Print and shaded views of the part. All mm, measured from the part's lowest x, y and z. A direction names the side the tool comes from. Round coordinates to 2 decimals unless told otherwise and drop trailing zeros. Loops run counter-clockwise (first coordinate to the right, second up) from the corner with the lowest first, then second, coordinate; pieces in that order, holes last. Notation, with made-up numbers: (72.25, 25.5) - (100.25, 25.5) arc R17 cw to (100.25, 45.5) - close; hole circle Ø3 at (48.25, 83). An arc over 180 degrees is marked (long way). Use one line per item in the form item = value. Start each with the question number.
Q1. Saw through at D-D (z = 5.25). Give the cut face in (x, y), then the cut area to 3 significant figures.
Q2. Pin check, flat tips, straight feed: pin 1 (4 mm diameter, centred on y = 8.5, z = 6, fed in from +X); pin 2 (1 mm diameter, centred on x = 9.5, z = 11.5, fed in from +Y). Stop position of each tip, or through.
Q3. Drill centre lines: line 1 (Y direction, x = 0.35, z = 7.5); line 2 (Y direction, x = 12.75, z = 1.5). Where is each one in solid material? Low to high.
Q4. 3-axis set-ups, long thin cutter, end or side, ignore diameter. For the marked faces 1 and 2: which of +Z, -Z, +X, -X, +Y, -Y reach the whole face in a straight line?
Q5. Saw through at A-A (y = 7.5). Give the cut face in (x, z), then the cut area to 3 significant figures.
Q6. Saw through at B-B (z = 7.5). Give the cut face in (x, y).
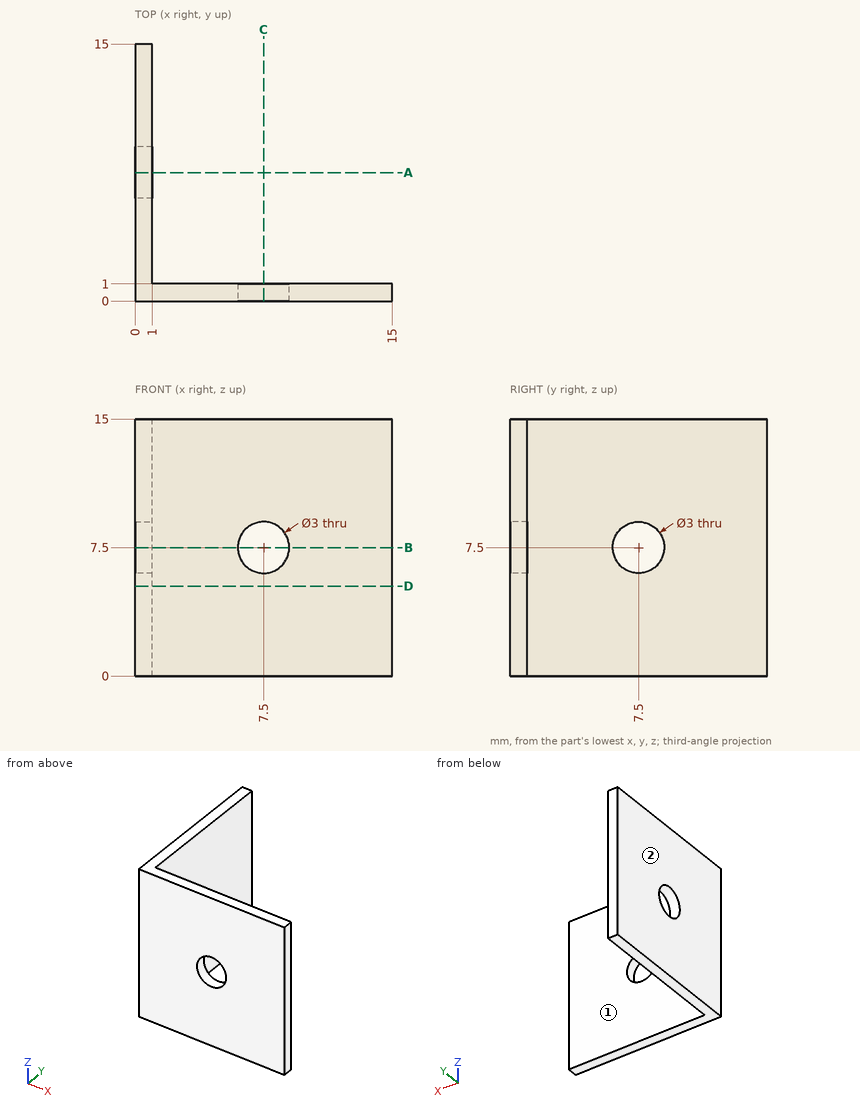
Report:
q1.outline = (0, 0) - (15, 0) - (15, 1) - (1, 1) - (1, 15) - (0, 15) - close
q1.area = 29.0 mm²
q2.pin_1 = 1
q2.pin_2 = 1
q3.line_1 = 0 to 6, 9 to 15
q3.line_2 = 0 to 1
q4.face_1 = +Z, -Z, +X, +Y
q4.face_2 = +Z, -Z, -X, +Y, -Y
q5.outline = (0, 0) - (1, 0) - (1, 6) - (0, 6) - close; (0, 9) - (1, 9) - (1, 15) - (0, 15) - close
q5.area = 12.0 mm²
q6.outline = (0, 0) - (6, 0) - (6, 1) - (1, 1) - (1, 6) - (0, 6) - close; (0, 9) - (1, 9) - (1, 15) - (0, 15) - close; (9, 0) - (15, 0) - (15, 1) - (9, 1) - close
